Read the model definition and answer for the solid it produces. Units are mm, in the model's axes. Round coordinates to 2 decimals unless told otherwise and drop trailing zeros. Loops run counter-clockwise (first coordinate to the right, second up) from the corner with the lowest first, then second, coordinate; pieces in that order, holes last. Notation, with made-up numbers: (87, 63) - (120, 63) arc R13 cw to (120, 74) - close; hole circle Ø4 at (12.25, -11). An arc over 180 degrees is marked (long way). Use CSV: the item, a comma, the result in double quotes. Start each with the question number.
1. Find section A-A (y = 12.7). Give the vertices of the cut face in (x, z) (3 decimals), and give its area (3 significant figures).
2. Find section C-C (x = 66.04). Give the vertices of the cut face in (y, z).
3. Given pin 1 Ø5.5 at (x, y) = (-33.02, 31.75) entering from +Z, flat-ended and moving along its own axis, determine where the tip first touches the part or whether it passes through.
4. Consider line 1 along Y through (x, z) = (33.02, 3.25); line 2 along Y through (x, z) = (65, 3); line 3 along X through (y, z) = (12, 0.75) (3 decimals). Determine where each line is inside the solid, lowest interval first.
5. Determine the mould class of faces 1 (the cylindrical face through (-33.488, 29.642, 3.131)), 2 (the cylindrical face through (120.006, -34.478, 3.219)), 3 (the flat face through (-2, 38.1, 3)), 4 (the cylindrical face through (-98.064, 29.835, 3.131)) for opening direction X: +X half, -X half, draft (parallel to the pull), parting line (faces both ways), or undercut.
6. Find section B-B (z = 3). State how many separate pieces and enclosed holes the cut face has, and give its area (3 significant figures).
from build123d import *

# Parameters (mm, degrees)
SKETCH1_W           = 247.65
SKETCH1_H           = 76.2
SKETCH1_R           = 2.159
BOSS_EXTRUDE1_DEPTH = 6.35
FILLET1_R           = 12.7


with BuildPart() as part:
    # Sketch1 → Boss-Extrude1 (new body)
    with BuildSketch(Plane.XY):
        Rectangle(SKETCH1_W, SKETCH1_H)
        with Locations((-117.475, 12.7)):
            Circle(SKETCH1_R, mode=Mode.SUBTRACT)
        with Locations((-117.475, -12.7)):
            Circle(SKETCH1_R, mode=Mode.SUBTRACT)
        with Locations((-99.06, -31.75)):
            Circle(SKETCH1_R, mode=Mode.SUBTRACT)
        with Locations((-66.04, -31.75)):
            Circle(SKETCH1_R, mode=Mode.SUBTRACT)
        with Locations((-33.02, -31.75)):
            Circle(SKETCH1_R, mode=Mode.SUBTRACT)
        with Locations((0, -31.75)):
            Circle(SKETCH1_R, mode=Mode.SUBTRACT)
        with Locations((33.02, -31.75)):
            Circle(SKETCH1_R, mode=Mode.SUBTRACT)
        with Locations((66.04, -31.75)):
            Circle(SKETCH1_R, mode=Mode.SUBTRACT)
        with Locations((99.06, -31.75)):
            Circle(SKETCH1_R, mode=Mode.SUBTRACT)
        with Locations((117.475, -12.7)):
            Circle(SKETCH1_R, mode=Mode.SUBTRACT)
        with Locations((117.475, 12.7)):
            Circle(SKETCH1_R, mode=Mode.SUBTRACT)
        with Locations((99.06, 31.75)):
            Circle(SKETCH1_R, mode=Mode.SUBTRACT)
        with Locations((66.04, 31.75)):
            Circle(SKETCH1_R, mode=Mode.SUBTRACT)
        with Locations((33.02, 31.75)):
            Circle(SKETCH1_R, mode=Mode.SUBTRACT)
        with Locations((0, 31.75)):
            Circle(SKETCH1_R, mode=Mode.SUBTRACT)
        with Locations((-33.02, 31.75)):
            Circle(SKETCH1_R, mode=Mode.SUBTRACT)
        with Locations((-66.04, 31.75)):
            Circle(SKETCH1_R, mode=Mode.SUBTRACT)
        with Locations((-99.06, 31.75)):
            Circle(SKETCH1_R, mode=Mode.SUBTRACT)
    extrude(amount=BOSS_EXTRUDE1_DEPTH)

    # Fillet1
    fillet1_edges = [part.edges().sort_by_distance(p)[0] for p in [
        (123.825, -38.1, 3.175),
        (-123.825, -38.1, 3.175),
    ]]
    fillet(fillet1_edges, radius=FILLET1_R)


solid = part.part
Filled sheet:
1,outline,"(-123.825, 0) - (-119.634, 0) - (-119.634, 6.35) - (-123.825, 6.35) - close; (-115.316, 0) - (115.316, 0) - (115.316, 6.35) - (-115.316, 6.35) - close; (119.634, 0) - (123.825, 0) - (123.825, 6.35) - (119.634, 6.35) - close"
1,area,"1,520 mm²"
2,outline,"(-38.1, 0) - (-33.91, 0) - (-33.91, 6.35) - (-38.1, 6.35) - close; (-29.59, 0) - (29.59, 0) - (29.59, 6.35) - (-29.59, 6.35) - close; (33.91, 0) - (38.1, 0) - (38.1, 6.35) - (33.91, 6.35) - close"
3,pin 1,"stops at z = 6.35"
4,line 1,"y = -38.1 to -33.91, -29.59 to 29.59, 33.91 to 38.1"
4,line 2,"y = -38.1 to -33.64, -29.86 to 29.86, 33.64 to 38.1"
4,line 3,"x = -123.825 to -119.517, -115.433 to 115.433, 119.517 to 123.825"
5,face 1,"undercut"
5,face 2,"+X half"
5,face 3,"draft"
5,face 4,"undercut"
6,separate pieces,"1"
6,enclosed holes,"18"
6,area,"18,500 mm²"
